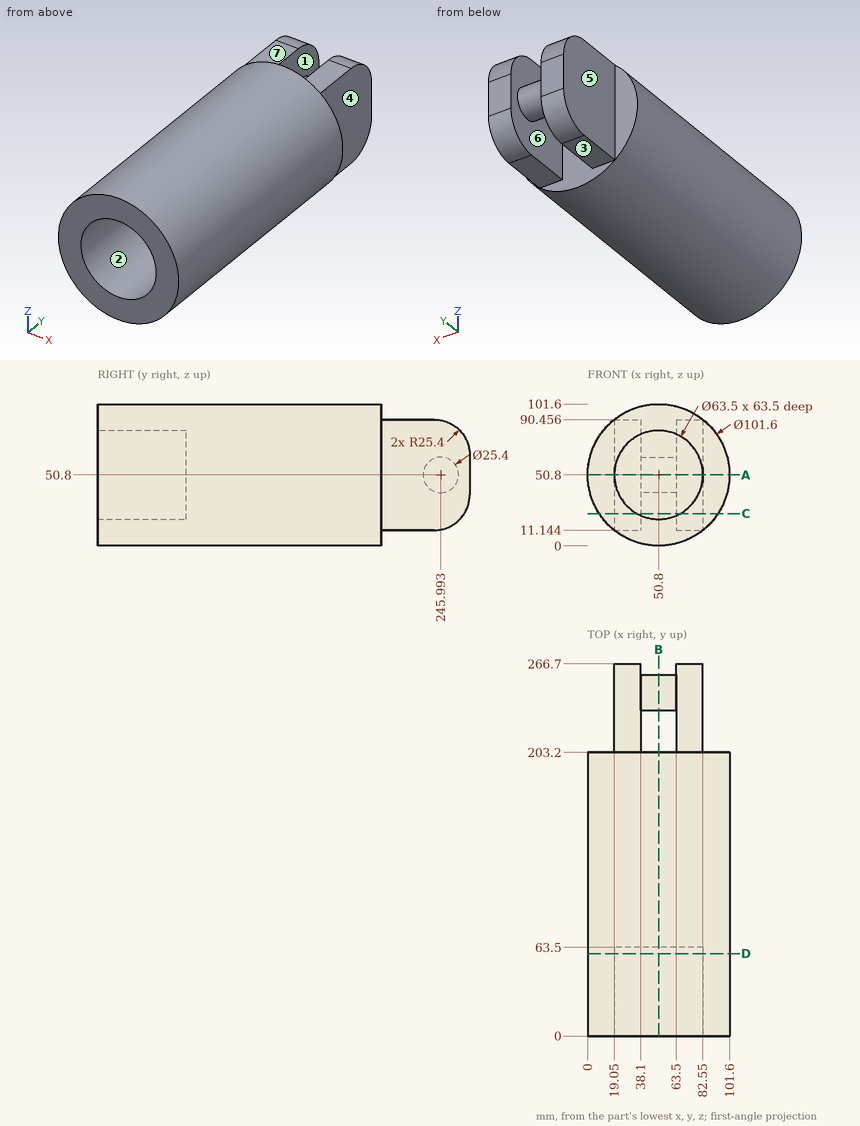
The figure shows three views and two pictorial views of one solid part (mm, origin at its lowest corner). Answer the questions. A direction names the side the tool comes from. Give positions to 0.01 mm unless a question says otherwise; leave off trailing zeros. Write each loop counter-clockwise with the first axis right and the second up, starting at its lowest first coordinate (ties: lowest second). Pieces come first, ordered by that corner, then holes. Notation, with made-up numbers: M 26.5,-36 L 66.5,-36 A20 cw 66.5,-17 Z; hole C 22,46 d10. An arc over 180 degrees is marked long. One line per item, written item: value. Start each with the question number.
(1) A tool of negligible diameter and unlimited length cuts with its end or side. For the marked faces 1, 2, 3 and 4, from which of +Z, -Z, +X, -X, +Y, -Y can it reach the whole face along a straight path? Write none if from no direction.
(2) Find section A-A (z = 50.8). Determine the outline of the cut face in (x, y), plus the area to 3 significant figures.
(3) Find section C-C (z = 23). Determine the outline of the cut face in (x, y), plus the area to 3 significant figures.
(4) Determine the mould class of the marked faces 5, 6 and 7 for opening direction X: pulls with the +X half, pulls with the -X half, needs draft (parallel to the pull), parting line crosses it, or undercut.
(5) Find the intervals of material crossed by line 1 (X direction, y = 48.5, z = 50.8); line 2 (X direction, y = 223.5, z = 61); line 3 (Y direction, x = 73.5, z = 41), in increasing order.
(6) Find section B-B (x = 50.8). Determine the outline of the cut face in (y, z).
(7) Find section D-D (y = 59). Determine the outline of the cut face in (x, z), plus the area to 3 significant figures.
(8) Flat-ended cylindrical pins translate along their axes: pin 1 Ø21 at (x, z) = (90.5, 39.5) entering from +Y; pin 2 Ø4 at (y, z) = (154, 78.5) entering from +X; pin 3 Ø9.5 at (x, y) = (74.5, 221) entering from +Z; pin 4 Ø10 at (y, z) = (235, 19) entering from +X. Find the tip coordinate at first contact, or state that the pin passes through.
Results below:
1. face 1: none
1. face 2: -Y
1. face 3: -Z, +X, -X, +Y
1. face 4: +Z, -Z, +X, +Y
2. outline: M 0,0 L 19.05,0 L 19.05,63.5 L 82.55,63.5 L 82.55,0 L 101.6,0 L 101.6,203.2 L 82.55,203.2 L 82.55,266.7 L 63.5,266.7 L 63.5,258.69 L 38.1,258.69 L 38.1,266.7 L 19.05,266.7 L 19.05,203.2 L 0,203.2 Z; hole M 38.1,203.2 L 63.5,203.2 L 63.5,233.29 L 38.1,233.29 Z
2. area: 19,700 mm^2
3. outline: M 8.28,0 L 35.46,0 L 35.46,63.5 L 66.14,63.5 L 66.14,0 L 93.32,0 L 93.32,203.2 L 82.55,203.2 L 82.55,262.79 L 63.5,262.79 L 63.5,203.2 L 38.1,203.2 L 38.1,262.79 L 19.05,262.79 L 19.05,203.2 L 8.28,203.2 Z
3. area: 17,600 mm^2
4. face 5: pulls with the -X half
4. face 6: undercut
4. face 7: needs draft
5. line 1: x = 0 to 19.05, 82.55 to 101.6
5. line 2: x = 19.05 to 38.1, 63.5 to 82.55
5. line 3: y = 63.5 to 266.7
6. outline: M 0,0 L 203.2,0 L 203.2,101.6 L 0,101.6 L 0,82.55 L 63.5,82.55 L 63.5,19.05 L 0,19.05 Z; C 245.99,50.8 d25.4
7. outline: C 50.8,50.8 d101.6; hole C 50.8,50.8 d63.5
7. area: 4,940 mm^2
8. pin 1: stops at y = 266.7
8. pin 2: stops at x = 94.62
8. pin 3: stops at z = 90.46
8. pin 4: stops at x = 82.55
